Could you check a few things on this model? Use its own coordinates, in mm. Face numbers are marked on the shaded views. A direction names the side the tool comes from. Coordinates: 2 decimals unless noted, no trailing zeros. Loops run counter-clockwise (first coordinate to the right, second up) from the corner with the lowest first, then second, coordinate; pieces in that order, holes last.
1) If I drill on line 1 along X through (y, z) = (3.6, 0); line 2 along Z through (x, y) = (0, 8.8) (3 decimals), over which ranges is the centre line in solid material (lowest first)?
2) Imagine slicing it at D-D on y = 6. Please give me the cut outline in (x, z) (3 decimals).
3) Imagine slicing it at A-A on z = 0. Please give me the cut outline in (x, y) (3 decimals).
4) Imagine slicing it at B-B on x = 0. Please give me the cut outline in (y, z) (3 decimals).
5) Thinking about a two-plate mould opening in X: for the marked faces 1, 2 and 3, which applies, released by +X, released by -X, zero draft, split by the parting line, or undercut?
6) Will these pins go through, and if not, where does the flat tip stop? P1, Ø2, axis at y = 6, z = -1, coming from the +X side; P2, Ø19, axis at x = 0, z = 0, coming from the -Y side; P3, Ø5, axis at y = -1, z = -3.5, coming from the +X side.
7) For the marked faces 4, 5 and 6, which set-ups out of +Z, -Z, +X, -X, +Y, -Y let a thin tool reach every point of the face, with its end or its side?
8) Imagine slicing it at C-C on z = -7.5. Please give me the cut outline in (x, y), plus the area to 3 significant figures.
Autodesk Inventor part; units mm, degrees
ref_plane "YZ Plane" through (0, 0, 0) normal (1, 0, 0) x (0, 1, 0)
ref_plane "XZ Plane" through (0, 0, 0) normal (0, 1, 0) x (-1, 0, 0)
ref_plane "XY Plane" through (0, 0, 0) normal (0, 0, 1) x (1, 0, 0)
sketch "Sketch1" plane through (0, 0, 0) normal (0, 1, 0) x (-1, 0, 0)
  circle A0 centre (0, 0) radius 12.7
  dimension "d1" = 25.4
extrude "Extrusion3" add sketch "Sketch1" along normal blind 5.08
sketch "Sketch3" plane through (0, 0, 0) normal (0, -1, 0) x (1, 0, 0)
  circle A0 centre (0, 0) radius 0.4685
hole "Hole1" at (0, 0, 0) direction (0, 1, 0) diameter 5.08 end through all counterbore diameter 38.1 counterbore depth 2.54
sketch "Sketch4" plane through (0, 2.54, 0) normal (0, -1, 0) x (1, 0, 0)
  circle A0 centre (0, 0) radius 11.9796
  circle A1 centre (0, 0) radius 19.05
  circle A2 centre (0, 0) radius 15.8934
extrude "Extrusion4" add sketch "Sketch4" along normal blind 5.08 contours A2
sketch "Sketch5" plane through (0, 5.08, 0) normal (0, 1, 0) x (1, 0, 0)
  point P0 (0, 0)
sketch "Sketch6" plane through (0, 5.08, 0) normal (0, 1, 0) x (1, 0, 0)
  circle A0 centre (0, 0) radius 5.08
  dimension "d19" = 10.16
sketch "Sketch7" plane through (0, 5.08, 0) normal (0, 1, 0) x (1, 0, 0)
  circle A0 centre (0, 0) radius 1.905
  dimension "d24" = 3.81
extrude "Extrusion5" add sketch "Sketch6" along normal blind 5.08
extrude "Extrusion6" cut sketch "Sketch7" along normal blind 5.08
properties part number "NEWWHEELS"
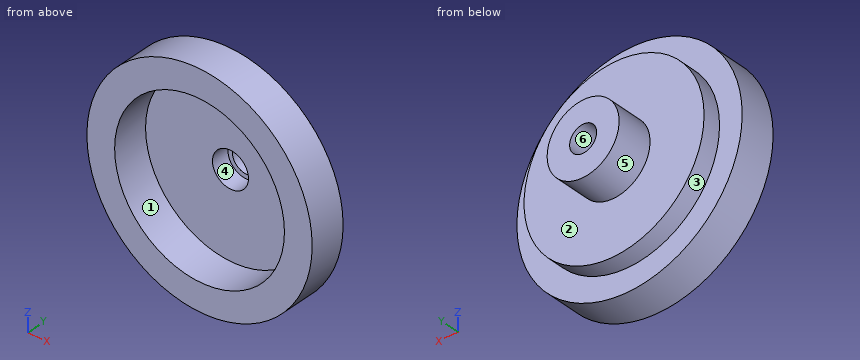
Filled in:
1. line 1: x = -12.7 to -2.54, 2.54 to 12.7
1. line 2: z = -5.08 to -1.905, 1.905 to 5.08
2. outline: circle Ø10.16 at (0, 0); hole circle Ø3.81 at (0, 0)
3. outline: (-15.893, -2.54) - (-11.98, -2.54) - (-11.98, 2.54) - (-2.54, 2.54) - (-2.54, 5.08) - (-1.905, 5.08) - (-1.905, 10.16) - (-5.08, 10.16) - (-5.08, 5.08) - (-12.7, 5.08) - (-12.7, 2.54) - (-15.893, 2.54) - close; (1.905, 5.08) - (2.54, 5.08) - (2.54, 2.54) - (11.98, 2.54) - (11.98, -2.54) - (15.893, -2.54) - (15.893, 2.54) - (12.7, 2.54) - (12.7, 5.08) - (5.08, 5.08) - (5.08, 10.16) - (1.905, 10.16) - close
4. outline: (-2.54, -15.893) - (2.54, -15.893) - (2.54, -12.7) - (5.08, -12.7) - (5.08, -5.08) - (10.16, -5.08) - (10.16, -1.905) - (5.08, -1.905) - (5.08, -2.54) - (2.54, -2.54) - (2.54, -11.98) - (-2.54, -11.98) - close; (-2.54, 11.98) - (2.54, 11.98) - (2.54, 2.54) - (5.08, 2.54) - (5.08, 1.905) - (10.16, 1.905) - (10.16, 5.08) - (5.08, 5.08) - (5.08, 12.7) - (2.54, 12.7) - (2.54, 15.893) - (-2.54, 15.893) - close
5. face 1: undercut
5. face 2: zero draft
5. face 3: split by the parting line
6. P1: stops at x = 12.69
6. P2: stops at y = 2.54
6. P3: stops at x = 15.86
7. face 4: -Y
7. face 5: +Y
7. face 6: +Y, -Y
8. outline: (-14.01, -2.54) - (-9.34, -2.54) - (-9.34, 2.54) - (9.34, 2.54) - (9.34, -2.54) - (14.01, -2.54) - (14.01, 2.54) - (10.25, 2.54) - (10.25, 5.08) - (-10.25, 5.08) - (-10.25, 2.54) - (-14.01, 2.54) - close
8. area: 99.5 mm2
